```python
from build123d import *

# Parameters (mm, degrees)
PAD_DEPTH            = 6.5
POCKET_DEPTH         = 6
SKETCH002_R          = 13.5
POCKET001_DEPTH      = 1
SKETCH003_W          = 5.4
SKETCH003_H          = 6.5
PAD001_DEPTH         = 3.5
POCKET002_DEPTH      = 10
SKETCH010_W          = 3.95
SKETCH010_H          = 6.5
PAD002_DEPTH         = 3.5
POCKET005_DEPTH      = 10
SKETCH015_R          = 2.2
SKETCH015_R_2        = 1.025
PAD003_DEPTH         = 2
POCKET009_DEPTH      = 4
POCKET010_DEPTH      = 4
PAD004_DEPTH         = 4
POCKET013_DEPTH      = 12.151
POCKET013_DEPTH_BACK = 36.251
SKETCH022_R          = 0.6
POCKET014_DEPTH      = 2
SKETCH023_R          = 0.6
POCKET015_DEPTH      = 2
SKETCH024_R          = 13.5
PAD005_DEPTH         = 0.5
SKETCH025_R          = 20.45
SKETCH025_R_2        = 19.85
POCKET016_DEPTH      = 0.3


with BuildPart() as part:
    # Sketch → Pad (new body)
    with BuildSketch(Plane.XY):
        with BuildLine():
            Line((-22.5019915649, 16), (-22.5019915649, -16))
            Line((-22.5019915649, -16), (-16.2858834578, -17.9))
            ThreePointArc((-16.2858834578, -17.9), (-0.4552796053, -24.1957169863), (15.6009615088, -18.5))
            Line((15.6009615088, -18.5), (24.5395016581, -17.45))
            Line((24.5395016581, 17.45), (24.5395016581, -17.45))
            Line((15.6009615088, 18.5), (24.5395016581, 17.45))
            ThreePointArc((15.6009615088, 18.5), (-0.4552796053, 24.1957169863), (-16.2858834578, 17.9))
            Line((-22.5019915649, 16), (-16.2858834578, 17.9))
        make_face()
    extrude(amount=PAD_DEPTH)

    # Sketch001 → Pocket (cut)
    with BuildSketch(Plane.XY):
        with BuildLine():
            Line((-14.8539557021, 16.9), (-21.2122180433, 15.55))
            Line((-21.2122180433, 15.55), (-21.2122180433, -15.55))
            Line((-21.2122180433, -15.55), (-14.8539557021, -16.9))
            ThreePointArc((-14.8539557021, -16.9), (-0.0760301383, -22.4998715423), (14.739402973, -17))
            Line((14.739402973, -17), (23.6191552218, -16.4))
            Line((23.6191552218, 16.4), (23.6191552218, -16.4))
            Line((14.739402973, 17), (23.6191552218, 16.4))
            ThreePointArc((14.739402973, 17), (-0.0760301383, 22.4998715423), (-14.8539557021, 16.9))
        make_face()
    extrude(amount=POCKET_DEPTH, mode=Mode.SUBTRACT)

    # Sketch002 (on Face19 of Pocket) → Pocket001 (cut)
    with BuildSketch(Plane(origin=(0, 0, 6), x_dir=(1, 0, 0), z_dir=(0, 0, -1))):
        Circle(SKETCH002_R)
    extrude(amount=-POCKET001_DEPTH, mode=Mode.SUBTRACT)

    # Sketch003 (on Face7 of Pad) → Pad001 (join)
    with BuildSketch(Plane.YZ.offset(24.5395016581)):
        with Locations((-14.75, 3.25)):
            Rectangle(SKETCH003_W, SKETCH003_H)
        with Locations((14.75, 3.25)):
            Rectangle(SKETCH003_W, SKETCH003_H)
    extrude(amount=PAD001_DEPTH)

    # Sketch006 (on Face22 of Pad001) → Pocket002 (cut)
    with BuildSketch(Plane.XY.offset(6.5)):
        with BuildLine():
            ThreePointArc((24.5395016581, 17.45), (26.1592830786, 16.2095505764), (28.0395016581, 15.4176006311))
            Line((28.0395016581, 17.45), (28.0395016581, 15.4176006311))
            Line((28.0395016581, 17.45), (24.5395016581, 17.45))
        make_face()
        with BuildLine():
            ThreePointArc((28.0395016581, -15.4176006311), (26.1592830786, -16.2095505765), (24.5395016581, -17.4500000001))
            Line((28.0395016581, -17.45), (24.5395016581, -17.45))
            Line((28.0395016581, -15.4176006311), (28.0395016581, -17.45))
        make_face()
    extrude(amount=-POCKET002_DEPTH, mode=Mode.SUBTRACT)

    # Sketch010 (on Face3 of Pad) → Pad002 (join)
    with BuildSketch(Plane(origin=(-22.5019915649, 0, 0), x_dir=(0, -1, 0), z_dir=(-1, 0, 0))):
        with Locations((-14.025, 3.25)):
            Rectangle(SKETCH010_W, SKETCH010_H)
        with Locations((14.025, 3.25)):
            Rectangle(SKETCH010_W, SKETCH010_H)
    extrude(amount=PAD002_DEPTH)

    # Sketch011 (on Face28 of Pad002) → Pocket005 (cut)
    with BuildSketch(Plane.XY.offset(6.5)):
        Polygon((-26.0019915649, 16), (-22.5019915649, 16), (-26.0019915649, 14.5), align=None)
        Polygon((-22.5019915649, -16), (-26.0019915649, -14.5), (-26.0019915649, -16), align=None)
    extrude(amount=-POCKET005_DEPTH, mode=Mode.SUBTRACT)

    # Sketch015 (on Face19 of Pocket) → Pad003 (join)
    with BuildSketch(Plane(origin=(0, 0, 6), x_dir=(1, 0, 0), z_dir=(0, 0, -1))):
        with Locations((-18.42, 13.32)):
            Circle(SKETCH015_R)
        with Locations((-18.42, 13.32)):
            Circle(SKETCH015_R_2, mode=Mode.SUBTRACT)
        with Locations((7.27, 18.56)):
            Circle(SKETCH015_R)
        with Locations((7.27, 18.56)):
            Circle(SKETCH015_R_2, mode=Mode.SUBTRACT)
        with Locations((5.37, -19.79)):
            Circle(SKETCH015_R)
        with Locations((5.37, -19.79)):
            Circle(SKETCH015_R_2, mode=Mode.SUBTRACT)
        with Locations((-18.42, -13.32)):
            Circle(SKETCH015_R)
        with Locations((-18.42, -13.32)):
            Circle(SKETCH015_R_2, mode=Mode.SUBTRACT)
    extrude(amount=PAD003_DEPTH)

    # Sketch016 (on Face4 of Pocket) → Pocket009 (cut)
    with BuildSketch(Plane(origin=(0, 0, 0), x_dir=(1, 0, 0), z_dir=(0, 0, -1))):
        with BuildLine():
            Line((-4.9992330338, 23.6779996848), (-5.0007669662, 21.9372361465))
            ThreePointArc((5.0007669662, 21.9372361465), (0, 22.5), (-5.0007669662, 21.9372361465))
            Line((5.0007669662, 23.6776757675), (5.0007669662, 21.9372361465))
            ThreePointArc((5.0007669662, 23.6776757675), (0.00078388, 24.1999999873), (-4.9992330338, 23.6779996848))
        make_face()
    extrude(amount=-POCKET009_DEPTH, mode=Mode.SUBTRACT)

    # Sketch017 (on Face4 of Pocket) → Pocket010 (cut)
    with BuildSketch(Plane(origin=(0, 0, 0), x_dir=(1, 0, 0), z_dir=(0, 0, -1))):
        with BuildLine():
            ThreePointArc((-3.2541322314, -22.2634369184), (0, -22.5), (3.2541322314, -22.2634369184))
            Line((3.2541322314, -22.2634369184), (3.5, -23.9455632634))
            ThreePointArc((-3.5, -23.9455632634), (0, -24.2), (3.5, -23.9455632634))
            Line((-3.2541322314, -22.2634369184), (-3.5, -23.9455632634))
        make_face()
        with BuildLine():
            ThreePointArc((-13.9498796389, -17.6536358312), (-11.25, -19.4855715851), (-8.3135572795, -20.9077680626))
            Line((-8.3135572795, -20.9077680626), (-8.9416927184, -22.487466094))
            ThreePointArc((-15.0038705449, -18.987466094), (-12.1, -20.9578147716), (-8.9416927184, -22.487466094))
            Line((-13.9498796389, -17.6536358312), (-15.0038705449, -18.987466094))
        make_face()
        with BuildLine():
            ThreePointArc((8.3135572795, -20.9077680626), (11.25, -19.4855715851), (13.9498796389, -17.6536358312))
            Line((13.9498796389, -17.6536358312), (15.0038705449, -18.987466094))
            ThreePointArc((8.9416927184, -22.487466094), (12.1, -20.9578147716), (15.0038705449, -18.987466094))
            Line((8.3135572795, -20.9077680626), (8.9416927184, -22.487466094))
        make_face()
    extrude(amount=-POCKET010_DEPTH, mode=Mode.SUBTRACT)

    # Sketch018 (on Face8 of Pocket005) → Pad004 (join)
    with BuildSketch(Plane(origin=(0, 0, 0), x_dir=(1, 0, 0), z_dir=(0, 0, -1))):
        Polygon((-26.0019915649, 14.5), (-26.0019915649, 12.05), (-22.5019915649, 12.05), (-22.5019915649, 16), align=None)
        Polygon((-26.0019915649, -12.05), (-22.5019915649, -12.05), (-22.5019915649, -16), (-26.0019915649, -14.5), align=None)
        with BuildLine():
            Line((24.5395016581, 17.4500000001), (24.5395016581, 12.05))
            Line((28.0395016581, 12.05), (24.5395016581, 12.05))
            Line((28.0395016581, 15.4176006311), (28.0395016581, 12.05))
            ThreePointArc((24.5395016581, 17.4500000001), (26.1592830786, 16.2095505765), (28.0395016581, 15.4176006311))
        make_face()
        with BuildLine():
            Line((24.5395016581, -12.05), (24.5395016581, -17.45))
            ThreePointArc((28.0395016581, -15.4176006311), (26.1592830786, -16.2095505764), (24.5395016581, -17.45))
            Line((28.0395016581, -12.05), (28.0395016581, -15.4176006311))
            Line((24.5395016581, -12.05), (28.0395016581, -12.05))
        make_face()
    extrude(amount=PAD004_DEPTH)

    # Sketch021 (on Face50 of Pad004) → Pocket013 (cut, two sides)
    with BuildSketch(Plane(origin=(0, -12.05, 0), x_dir=(-1, 0, 0), z_dir=(0, 1, 0))) as pocket013_sk:
        with BuildLine():
            Line((-24.5395016581, -4), (-24.5395016581, -2))
            ThreePointArc((-26.5395016581, -4), (-25.1252880957, -3.4142135624), (-24.5395016581, -2))
            Line((-24.5395016581, -4), (-26.5395016581, -4))
        make_face()
        with BuildLine():
            Line((22.5019915649, -4), (22.5019915649, -2))
            ThreePointArc((22.5019915649, -2), (23.0877780026, -3.4142135624), (24.5019915649, -4))
            Line((22.5019915649, -4), (24.5019915649, -4))
        make_face()
        with BuildLine():
            Line((-28.0395016581, 0), (-28.0395016581, 6.5))
            Line((-28.0395016581, 6.5), (-24.5395016581, 6.5))
            ThreePointArc((-24.5395016581, 6.5), (-27.1088837932, 3.6912057651), (-28.0395016581, 0))
        make_face()
        with BuildLine():
            Line((26.0019915649, 6.5), (26.0019915649, 0))
            ThreePointArc((26.0019915649, 0), (25.0713737, 3.6912057651), (22.5019915649, 6.5))
            Line((26.0019915649, 6.5), (22.5019915649, 6.5))
        make_face()
    extrude(amount=-POCKET013_DEPTH, mode=Mode.SUBTRACT)
    extrude(pocket013_sk.sketch, amount=POCKET013_DEPTH_BACK, mode=Mode.SUBTRACT)

    # Sketch022 (on Face66 of Pocket013) → Pocket014 (cut)
    with BuildSketch(Plane.XZ.offset(-12.05)):
        with Locations((-24.7019915649, -2.7)):
            Circle(SKETCH022_R)
        with Locations((26.7395016581, -2.7)):
            Circle(SKETCH022_R)
    extrude(amount=-POCKET014_DEPTH, mode=Mode.SUBTRACT)

    # Sketch023 (on Face49 of Pocket014) → Pocket015 (cut)
    with BuildSketch(Plane(origin=(0, -12.05, 0), x_dir=(-1, 0, 0), z_dir=(0, 1, 0))):
        with Locations((-26.7395016581, -2.7)):
            Circle(SKETCH023_R)
        with Locations((24.7019915649, -2.7)):
            Circle(SKETCH023_R)
    extrude(amount=-POCKET015_DEPTH, mode=Mode.SUBTRACT)

    # Sketch024 (on Face16 of Pocket015) → Pad005 (join)
    with BuildSketch(Plane.XY.offset(6.5)):
        with BuildLine():
            ThreePointArc((-22.5019915649, -8.9050758341), (24.2, 0), (-22.5019915649, 8.9050758341))
            Line((-22.5019915649, 8.9050758341), (-22.5019915649, -8.9050758341))
        make_face()
        Circle(SKETCH024_R, mode=Mode.SUBTRACT)
    extrude(amount=PAD005_DEPTH)

    # Sketch025 (on Face42 of Pad005) → Pocket016 (cut)
    with BuildSketch(Plane.XY.offset(7)):
        Circle(SKETCH025_R)
        Circle(SKETCH025_R_2, mode=Mode.SUBTRACT)
    extrude(amount=-POCKET016_DEPTH, mode=Mode.SUBTRACT)


solid = part.part
```
Here's how the part is built. I have some questions about the finished solid (model axes, mm). A direction names the side the tool comes from. Round coordinates to 2 decimals unless told otherwise and drop trailing zeros. Order: outer loops, then holes, each group sorted by start corner. A loop starts at its lowest first (then second) coordinate and runs counter-clockwise, first axis right, second up. Notation, with made-up numbers: M 43.25,76.5 L 95.25,76.5 A35 ccw 95.25,113.5 Z; hole C 2,-23.75 d8. An arc over 180 degrees is marked long. Answer in a Markdown table with one row per item.
Item 1: Imagine slicing it at C-C, the plane x = 11. Write out the boundary of the cut face in (y, z).
A:
| item | result |
|---|---|
| outline | M -21.56,0 L -19.63,0 L -19.63,6 L -7.83,6 L -7.83,7 L -16.52,7 L -16.52,6.7 L -17.24,6.7 L -17.24,7 L -21.56,7 Z; M 7.83,6 L 19.63,6 L 19.63,4 L 21.56,4 L 21.56,7 L 17.24,7 L 17.24,6.7 L 16.52,6.7 L 16.52,7 L 7.83,7 Z |
Item 2: Thinking about a two-plate mould opening in Y: for faces 1 (the face through (27, -14, -4)), 2 (the face through (4.61, 19.1, 5.01)), which applies, +Y half, -Y half, draft (parallel to the pull), parting line (faces both ways), or undercut?
A:
| item | result |
|---|---|
| face 1 | draft |
| face 2 | undercut |
Item 3: Imagine slicing it at B-B, the plane z = -2.7. State how many separate pieces and enclosed holes the cut face has, and give its area (3 significant figures).
A:
| item | result |
|---|---|
| separate pieces | 4 |
| enclosed holes | 0 |
| area | 39.7 mm2 |
Item 4: If I drill on L1, parallel to Y at x = 0, z = 6.85; L2, parallel to X at y = -18.56, z = 5.35 (3 decimals); L3, parallel to X at y = 19.79, z = 5.45 (3 decimals), over which ranges is the centre line in solid material (lowest first)? Write a range as from..to.
A:
| item | result |
|---|---|
| L1 | y = -24.2..-20.45, -19.85..-13.5, 13.5..19.85, 20.45..24.2 |
| L2 | x = -15.53..-12.719, 5.07..6.245, 8.295..9.47, 12.719..15.53 |
| L3 | x = -13.928..-10.705, 3.17..4.345, 6.395..7.57, 10.705..13.928 |
Item 5: I'm going to push flat-ended pins straight in: pin 1 (1.5 mm diameter, centred on y = 4.5, z = 1, fed in from +X); pin 2 (2.5 mm diameter, centred on x = -18.42, y = -13.32, fed in from -Z); pin 3 (5 mm diameter, centred on x = 14, z = 4, fed in from -Y). Where does each tip first touch, or does it pass through?
A:
| item | result |
|---|---|
| pin 1 | stops at x = 24.54 |
| pin 2 | stops at z = 4 |
| pin 3 | stops at y = -21.29 |
Item 6: Imagine slicing it at A-A, the plane x = 0. Write out the boundary of the cut face in (y, z), and give its area (3 significant figures).
A:
| item | result |
|---|---|
| outline | M -24.2,4 L -22.5,4 L -22.5,6 L -13.5,6 L -13.5,7 L -19.85,7 L -19.85,6.7 L -20.45,6.7 L -20.45,7 L -24.2,7 Z; M 13.5,6 L 22.5,6 L 22.5,4 L 24.2,4 L 24.2,7 L 20.45,7 L 20.45,6.7 L 19.85,6.7 L 19.85,7 L 13.5,7 Z |
| area | 27.8 mm2 |
Item 7: For faces 3 (the face through (-26.002, 13, -2)), 4 (the face through (11, -10, 6)), 5 (the face through (-21, -14, 6.5)), 6 (the face through (24.54, 15, -1)), which set-ups out of +Z, -Z, +X, -X, +Y, -Y let a thin tool reach every point of the face, with its end or its side?
A:
| item | result |
|---|---|
| face 3 | +Z, -Z, -X, +Y, -Y |
| face 4 | -Z |
| face 5 | +Z, -X, -Y |
| face 6 | -Z, +Y, -Y |
Item 8: Imagine slicing it at D-D, the plane x = 17. Write out the boundary of the cut face in (y, z), and give its area (3 significant figures).
A:
| item | result |
|---|---|
| outline | M -18.34,0 L -16.85,0 L -16.85,6 L 16.85,6 L 16.85,0 L 18.34,0 L 18.34,6.5 L 17.22,6.5 L 17.22,7 L 11.37,7 L 11.37,6.7 L 10.25,6.7 L 10.25,7 L -10.25,7 L -10.25,6.7 L -11.37,6.7 L -11.37,7 L -17.22,7 L -17.22,6.5 L -18.34,6.5 Z |
| area | 52.7 mm2 |
